from build123d import *

# Parameters (mm, degrees)
F0_W     = 177.8
F0_H     = 38.1
F1_DEPTH = 2133.6


with BuildPart() as f1:
    # F0 (on Right) → F1 (new body)
    with BuildSketch(Plane.YZ):
        Polygon((0, 38.1), (0, 0), (266.7, 0), (266.7, 88.9), (0, 88.9), align=None)
        with Locations((-88.9, 19.05)):
            Rectangle(F0_W, F0_H)
        Polygon((266.7, 88.9), (266.7, 0), (266.7, -88.9), (304.8, -88.9), (304.8, 88.9), align=None)
        Polygon((-444.5, 0), (-177.8, 0), (-177.8, 38.1), (-177.8, 88.9), (-444.5, 88.9), align=None)
        Polygon((-444.5, -88.9), (-444.5, 0), (-444.5, 88.9), (-482.6, 88.9), (-482.6, -88.9), align=None)
    extrude(amount=F1_DEPTH)


solid = f1.part
Build history of the part. All positions in model axes, mm. A direction names the side the tool comes from. Round coordinates to 2 decimals unless told otherwise and drop trailing zeros. Write each loop counter-clockwise with the first axis right and the second up, starting at its lowest first coordinate (ties: lowest second). Pieces come first, ordered by that corner, then holes. Notation, with made-up numbers: (19, -8) - (75, -8) arc R11 ccw to (75, 1) - close; hole circle Ø9 at (27, -25.5). An arc over 180 degrees is marked (long way). One line per question, with ' | ' between items.
1. Mould opens along Y. For faces 1 (the face through (1052, 304.8, -1)), 2 (the face through (1052, 266.7, -44)), 3 (the face through (2133.6, -94, 21)) say: released by +Y, released by -Y, zero draft, split by the parting line, or undercut.
Results are:
face 1: released by +Y | face 2: undercut | face 3: zero draft
2. Band-saw the part on C-C, the plane z = 58.5. Write the cut outline in (x, y), and give its area (3 significant figures).
Results are:
outline: (0, -482.6) - (2133.6, -482.6) - (2133.6, -177.8) - (0, -177.8) - close; (0, 0) - (2133.6, 0) - (2133.6, 304.8) - (0, 304.8) - close | area: 1,300,000 mm^2
3. Drop a flat-ended pin along its axis: pin 1 Ø8 at (x, y) = (1707, -331.5) entering from -Z. Give the stop position or say it passes through.
Results are:
pin 1: z = 0
4. Tool access for faces 4 (the face through (1052, -94, 0)), 5 (the face through (1052, 155, 88.9)), 6 (the face through (1052, -90, 38.1)): list every direction of +Z, -Z, +X, -X, +Y, -Y with a clear straight run to the whole face (end or side of a thin tool).
Results are:
face 4: -Z, +X, -X | face 5: +Z, +X, -X, +Y, -Y | face 6: +Z, +X, -X
5. Band-saw the part on B-B, the plane x = 287. Write the cut outline in (y, z), and give its area (3 significant figures).
Results are:
outline: (-482.6, -88.9) - (-444.5, -88.9) - (-444.5, 0) - (266.7, 0) - (266.7, -88.9) - (304.8, -88.9) - (304.8, 88.9) - (0, 88.9) - (0, 38.1) - (-177.8, 38.1) - (-177.8, 88.9) - (-482.6, 88.9) - close | area: 67,700 mm^2
6. Drill centre lines: line 1 along Y through (x, z) = (697.5, -36.5); line 2 along Z through (x, y) = (984.5, -266); line 3 along Z through (x, y) = (738, -45). Where is each one in solid material? Low to high. Write a range as from..to.
Results are:
line 1: -482.6..-444.5, 266.7..304.8 | line 2: 0..88.9 | line 3: 0..38.1
7. Band-saw the part on D-D, the plane y = -32.5. Write the cut outline in (x, z), and give its area (3 significant figures).
Results are:
outline: (0, 0) - (2133.6, 0) - (2133.6, 38.1) - (0, 38.1) - close | area: 81,300 mm^2
8. Band-saw the part on A-A, the plane z = -44.5. Write the cut outline in (x, y).
Results are:
outline: (0, -482.6) - (2133.6, -482.6) - (2133.6, -444.5) - (0, -444.5) - close; (0, 266.7) - (2133.6, 266.7) - (2133.6, 304.8) - (0, 304.8) - close
